Geometry check sheet. Reference: the model listing, model coordinates, mm. Face numbers are marked on the shaded views. Give positions to 0.01 mm unless a question says otherwise; leave off trailing zeros. Order: outer loops, then holes, each group sorted by start corner. A loop starts at its lowest first (then second) coordinate and runs counter-clockwise, first axis right, second up. Notation, with made-up numbers: M -23.5,32 L 11.5,32 A6 cw 11.5,39 Z; hole C 30,29.5 d4. An arc over 180 degrees is marked long. Answer as CSV lines item,"result". Start each with the question number.
Q1. Go/stop test with a flat-tipped pin: pin 1 (1 mm diameter, centred on x = -1.5, y = -23.5, fed in from -Z). Record where the tip stops, or that it passes through.
Q2. Section check B-B, the plane x = 0. Record the boundary of the cut face in (y, z), then the cut area to 3 significant figures.
Q3. Section check C-C, the plane z = 6.5. Record the boundary of the cut face in (x, y).
Q4. Thickness scan on line 1 (Y direction, x = 0, z = 6); line 2 (X direction, y = -6.5, z = 15); line 3 (X direction, y = -10, z = 4.75). Record the ranges inside material, lowest first.
Q5. Section check A-A, the plane y = 0. Record the boundary of the cut face in (x, z).
Q6. Mould release check, pull along Y, two halves, no side actions. Record for the marked faces 1, 2, 3 and 4: +Y half, -Y half, draft (parallel to the pull), parting line (faces both ways), or undercut.
```python
from build123d import *

# Parameters (mm, degrees)
F0_W     = 108.715884
F0_H     = 69.138416
F0_R     = 19.075382
F1_DEPTH = 25.4
F2_R     = 5.08


with BuildPart() as f1:
    # F0 (on Top) → F1 (new body)
    with BuildSketch(Plane.XY):
        Rectangle(F0_W, F0_H)
        Circle(F0_R, mode=Mode.SUBTRACT)
    extrude(amount=F1_DEPTH)

    # F2
    f2_edges = [f1.edges().sort_by_distance(p)[0] for p in [
        (0, -34.569208, 25.4),
        (-54.357942, 0, 25.4),
        (0, 34.569208, 25.4),
        (54.357942, 0, 25.4),
        (-19.075382, 0, 25.4),
    ]]
    fillet(f2_edges, radius=F2_R)


solid = f1.part
```
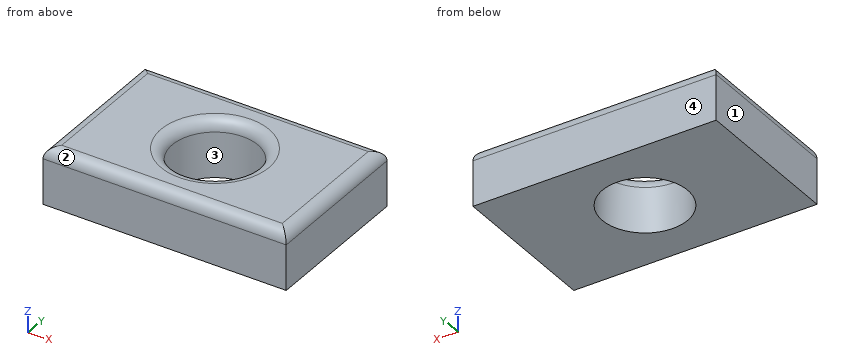
Answer block:
1,pin 1,"stops at z = 0"
2,outline,"M -34.57,0 L -19.08,0 L -19.08,20.32 A5.08 ccw -24.16,25.4 L -29.49,25.4 A5.08 ccw -34.57,20.32 Z; M 19.08,0 L 34.57,0 L 34.57,20.32 A5.08 ccw 29.49,25.4 L 24.16,25.4 A5.08 ccw 19.08,20.32 Z"
2,area,"765 mm2"
3,outline,"M -54.36,-34.57 L 54.36,-34.57 L 54.36,34.57 L -54.36,34.57 Z; hole C 0,0 d38.15"
4,line 1,"y = -34.57 to -19.08, 19.08 to 34.57"
4,line 2,"x = -54.36 to -17.93, 17.93 to 54.36"
4,line 3,"x = -54.36 to -16.24, 16.24 to 54.36"
5,outline,"M -54.36,0 L -19.08,0 L -19.08,20.32 A5.08 ccw -24.16,25.4 L -49.28,25.4 A5.08 ccw -54.36,20.32 Z; M 19.08,0 L 54.36,0 L 54.36,20.32 A5.08 ccw 49.28,25.4 L 24.16,25.4 A5.08 ccw 19.08,20.32 Z"
6,face 1,"draft"
6,face 2,"-Y half"
6,face 3,"undercut"
6,face 4,"+Y half"
